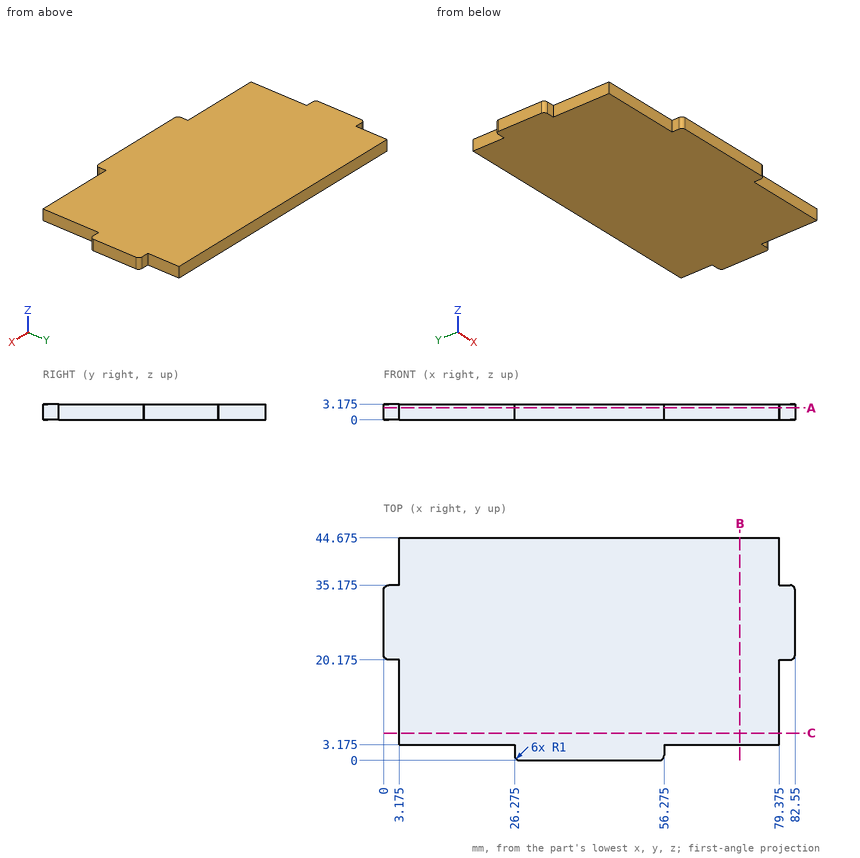
Answer from the drawing. Dimensions are ordinates in mm from the lowest x, y and z of the part. Give positions to 0.01 mm unless a question says otherwise; leave off trailing zeros. Order: outer loops, then holes, each group sorted by start corner. A loop starts at its lowest first (then second) coordinate and runs counter-clockwise, first axis right, second up. Notation, with made-up numbers: (46, 61) - (68, 61) arc R35 cw to (68, 95) - close; hole circle Ø8 at (40, 60). An arc over 180 degrees is marked (long way). Use one line per item in the form item = value.
1) Find section C-C on y = 5.5. Determine the outline of the cut face in (x, z) (3 decimals).
Verdict:
outline = (3.175, 0) - (79.375, 0) - (79.375, 3.175) - (3.175, 3.175) - close
2) Each of these flat-tipped pins is pushed along its axis until it touches: pin 1 (1.5 mm diameter, centred on x = 58.5, z = 2, fed in from -Y) (3 decimals); pin 2 (1.7 mm diameter, centred on y = 2.5, z = 1.5, fed in from -X) (3 decimals); pin 3 (1.7 mm diameter, centred on y = 1.5, z = 2, fed in from +X) (3 decimals). Where does it stop, or does it pass through?
Verdict:
pin_1 = 3.175
pin_2 = 3.175
pin_3 = 56.275
3) Consider probe 1 along X at (y, z) = (17.5, 2.55) (3 decimals); probe 2 along Y at (x, z) = (56.5, 0.6) (3 decimals). Determine where each line is inside the solid, lowest interval first. Write a range as [from, to].
Verdict:
probe_1 = [3.175, 79.375]
probe_2 = [3.175, 44.675]
4) Find section B-B on x = 71.5. Determine the outline of the cut face in (y, z) (3 decimals), and give its area (3 significant figures).
Verdict:
outline = (3.175, 0) - (44.675, 0) - (44.675, 3.175) - (3.175, 3.175) - close
area = 132 mm^2
5) Find section A-A on z = 2.4. Determine the outline of the cut face in (x, y) (3 decimals), and give its area (3 significant figures).
Verdict:
outline = (0, 21.175) arc R1 ccw to (1, 20.175) - (3.175, 20.175) - (3.175, 3.175) - (26.275, 3.175) - (26.275, 1) arc R1 ccw to (27.275, 0) - (55.275, 0) arc R1 ccw to (56.275, 1) - (56.275, 3.175) - (79.375, 3.175) - (79.375, 20.175) - (81.55, 20.175) arc R1 ccw to (82.55, 21.175) - (82.55, 34.175) arc R1 ccw to (81.55, 35.175) - (79.375, 35.175) - (79.375, 44.675) - (3.175, 44.675) - (3.175, 35.175) - (1, 35.175) arc R1 ccw to (0, 34.175) - close
area = 3,350 mm^2
